The model under review builds one solid part; all positions refer to its coordinate system, in mm. Round coordinates to 2 decimals unless told otherwise and drop trailing zeros. Loops run counter-clockwise (first coordinate to the right, second up) from the corner with the lowest first, then second, coordinate; pieces in that order, holes last. Notation, with made-up numbers: (9.5, -10.5) - (51.5, -10.5) arc R30 cw to (51.5, 18.5) - close; hole circle Ø3 at (33, -35.75). An arc over 180 degrees is marked (long way). Answer as CSV lines item,"result".
Autodesk Inventor part; units mm, degrees
ref_plane "YZ Plane" through (0, 0, 0) normal (1, 0, 0) x (0, 1, 0)
ref_plane "XZ Plane" through (0, 0, 0) normal (0, 1, 0) x (-1, 0, 0)
ref_plane "XY Plane" through (0, 0, 0) normal (0, 0, 1) x (1, 0, 0)
sketch "Sketch1" plane through (0, 0, 0) normal (0, 0, 1) x (1, 0, 0)
  circle A0 centre (-60, 36.0506) radius 2.75
  dimension "d1" = 5.5
extrude "Extrusion1" add sketch "Sketch1" along normal blind 2.7
fillet "Fillet1" radius 2 1 edges at (-62.75, 36.0506, 2.7)
sketch "Sketch4" plane through (-60, 36.0506, 0) normal (0, 0, -1) x (-1, 0, 0)
  circle A0 centre (0, 0) radius 2.75
  dimension "d11" = 5.5
extrude "Extrusion3" add sketch "Sketch4" along normal blind 2.7
properties part number "d-padball"
1. Clearance check with a flat-ended pin moving along its axis: pin 1 (1 mm diameter, centred on x = -61.5, z = 1, fed in from +Y). State where the tip first meets the part, or that it passes through.
Numbers:
pin 1,"stops at y = 38.6"
2. Wall thickness on probe 1 along Y at (x, z) = (-61.65, -2); probe 2 along Z at (x, y) = (-61.15, 37.7); probe 3 along X at (y, z) = (33.8, -1.35): over which ranges is each line inside the solid? List them lowest first.
Numbers:
probe 1,"y = 33.85 to 38.25"
probe 2,"z = -2.7 to 2.25"
probe 3,"x = -61.58 to -58.42"
3. Take a section at A-A (z = 0.5). State the section outline as (x, y) points.
Numbers:
outline,"circle Ø5.5 at (-60, 36.05)"
